Answer from the drawing. Dimensions are ordinates in mm from the lowest x, y and z of the part. Give positions to 0.01 mm unless a question says otherwise; leave off trailing zeros. Write each loop counter-clockwise with the first axis right and the second up, starting at its lowest first coordinate (ties: lowest second). Pieces come first, ordered by that corner, then holes. Notation, with made-up numbers: M 11,-31 L 21,-31 A17 ccw 21,-18 Z; hole C 39,81.25 d10. An arc over 180 degrees is marked long. Answer as a JSON object with one key per item and string values.
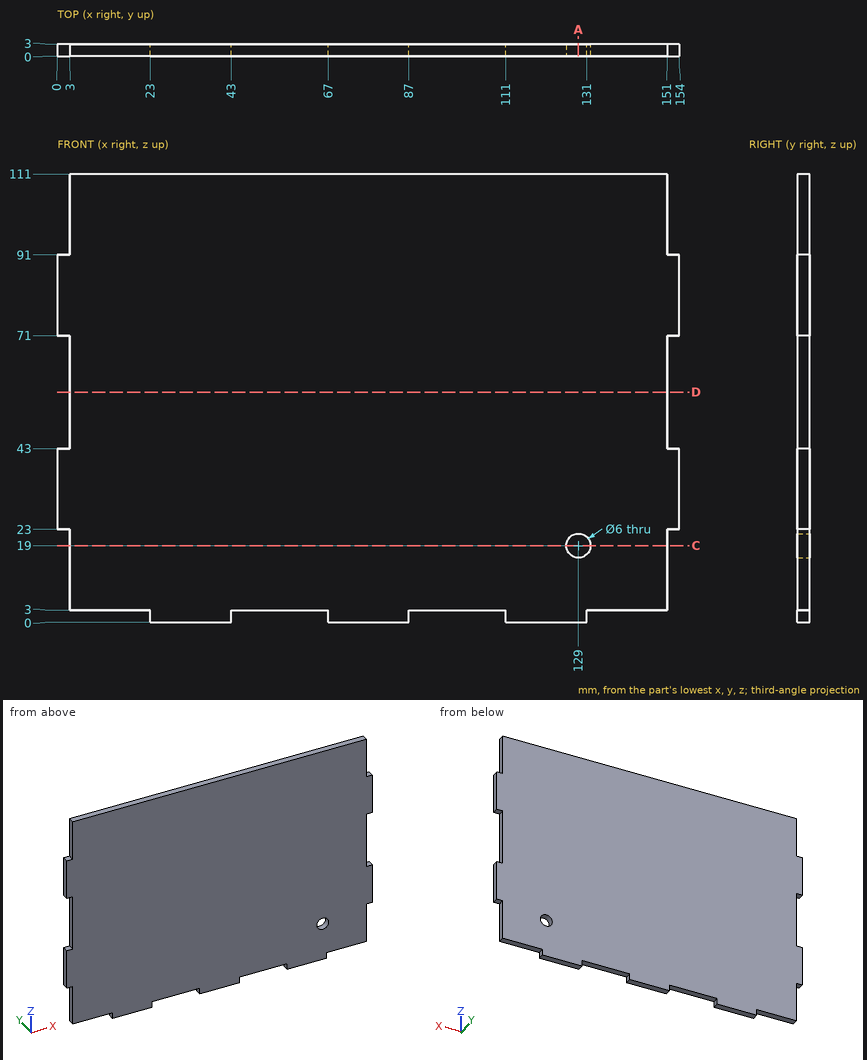
1. A cutting plane is placed at D-D, the plane z = 57. Give the vertices of the cut face in (x, y), plus the area to 3 significant figures.
Verdict:
{"outline": "M 3,0 L 151,0 L 151,3 L 3,3 Z", "area": "444 mm2"}
2. A cutting plane is placed at C-C, the plane z = 19. Give the vertices of the cut face in (x, y), plus the area to 3 significant figures.
Verdict:
{"outline": "M 3,0 L 126,0 L 126,3 L 3,3 Z; M 132,0 L 151,0 L 151,3 L 132,3 Z", "area": "426 mm2"}
3. Consider line 1 along Z through (x, y) = (129, 2.3); line 2 along X through (y, z) = (1.75, 94.5); line 3 along Z through (x, y) = (146, 1.35). Determine where each line is inside the solid, lowest interval first.
Verdict:
{"line 1": "z = 0 to 16, 22 to 111", "line 2": "x = 3 to 151", "line 3": "z = 3 to 111"}
4. A cutting plane is placed at A-A, the plane x = 129. Give the vertices of the cut face in (y, z), plus the area to 3 significant figures.
Verdict:
{"outline": "M 0,0 L 3,0 L 3,16 L 0,16 Z; M 0,22 L 3,22 L 3,111 L 0,111 Z", "area": "315 mm2"}
5. Flat-ended cylindrical pins translate along their axes: pin 1 (1 mm diameter, centred on y = 0.5, z = 59, fed in from +X); pin 2 (1.5 mm diameter, centred on x = 2, y = 2, fed in from -Z); pin 3 (0.9 mm diameter, centred on y = 2, z = 13, fed in from -X); pin 4 (5.5 mm diameter, centred on x = 129, z = 19, fed in from +Y). Find the tip coordinate at first contact, or state that the pin passes through.
Verdict:
{"pin 1": "stops at x = 151", "pin 2": "stops at z = 23", "pin 3": "stops at x = 3", "pin 4": "passes through"}
